For this review, take the finished solid that the model builds, in its own axes (mm). A direction names the side the tool comes from. Round coordinates to 2 decimals unless told otherwise and drop trailing zeros. Write each loop counter-clockwise with the first axis right and the second up, starting at its lowest first coordinate (ties: lowest second). Pieces come first, ordered by that corner, then holes. Notation, with made-up numbers: (68, 61.25) -> (91, 61.25) arc R12 ccw to (91, 68.25) -> close; hole circle Ø10 at (60, 75.25). An arc over 180 degrees is marked (long way). Answer as CSV lines item,"result". Start each with the question number.
Item 1: Take a section at C-C on y = 28. Give the boundary of the cut face in (x, z), then the cut area to 3 significant figures.
Item 2: Wall thickness on probe 1 along X at (y, z) = (23.5, -11.5); probe 2 along Y at (x, z) = (-25.5, 11.5); probe 3 along Z at (x, y) = (13, 22): over which ranges is each line inside the solid? List them lowest first. Write a range as from..to.
Item 3: Take a section at B-B on z = 19. Give the boundary of the cut face in (x, y), then the cut area to 3 significant figures.
Item 4: Take a section at A-A on z = -12.5. Give the boundary of the cut face in (x, y), then the cut area to 3 significant figures.
Item 5: Machinability: for faces 4 (the flat face through (-31, 2, -18.85)), 5 (the flat face through (-1, 5, -3)), 6 (the flat face through (18, 18, -16.85)), 7 (the flat face through (-1, 2, 21.15)), 8 (the cylindrical face through (-33.25, 2.54, 18.15)), which of the approach directions +Z, -Z, +X, -X, +Y, -Y give a long, thin tool a straight path to every point of the face, cutting with its end or side? Answer none if there is none.
Item 6: Take a section at D-D on x = -28. Give the boundary of the cut face in (y, z), then the cut area to 3 significant figures.
Item 7: For pin 1 Ø12 at (y, z) = (29, -4.5) entering from -X; pin 2 Ø13.5 at (y, z) = (20.5, -5) entering from +X; pin 3 Ø1.5 at (x, y) = (-7, 2.5) entering from +Z; pin 4 Ø6 at (y, z) = (20.5, -21) entering from +X, all flat-tipped, find the tip position at first contact; note any pin that passes through.
Item 8: Mouldability with a two-part tool opening along Z and no side actions: class faces 1 (the flat face through (31.289, 3, 1)), 2 (the flat face through (43.289, 2, 8)), 3 (the flat face through (-1, 20, 22.08)) as +Z half, -Z half, draft (parallel to the pull), parting line (faces both ways), or undercut.
```python
from build123d import *

# Parameters (mm, degrees)
EXTRUDE_1_DEPTH     = 5
SKETCH_4_W          = 1.8
SKETCH_4_H          = 37
EXTRUDE_2_DEPTH     = 27
SKETCH_5_W          = 40.5
SKETCH_5_H          = 37
EXTRUDE_3_DEPTH     = 3
CUT_EXTRUDE_4_DEPTH = 10
CUT_EXTRUDE_7_DEPTH = 10
CUT_EXTRUDE_8_DEPTH = 10
SKETCH_13_R         = 7.5
CUT_EXTRUDE_9_DEPTH = 10
SKETCH_14_W         = 40.5
SKETCH_14_H         = 30
EXTRUDE_4_DEPTH     = 2


with BuildPart() as part:
    # 草图1 → 凸台-拉伸1 (new body)
    with BuildSketch(Plane(origin=(0, 0, 0), x_dir=(1, 0, 0), z_dir=(0, 1, 0))):
        Polygon((13.545654436, 26.428234879), (-13.545654436, 26.428234879), (-19.229145808, 18.850246383), (-43.289259281, 18.850246383), (-43.289259281, -21.149753617), (43.289259281, -21.149753617), (43.289259281, 18.850246383), (19.229145808, 18.850246383), align=None)
    extrude(amount=EXTRUDE_1_DEPTH)

    # 草图4 → 凸台-拉伸2 (add)
    with BuildSketch(Plane(origin=(0, 5, 0), x_dir=(1, 0, 0), z_dir=(0, 1, 0))):
        with Locations((-20.389259281, -1.649753617)):
            Rectangle(SKETCH_4_W, SKETCH_4_H)
        with Locations((18.410740719, -1.649753617)):
            Rectangle(SKETCH_4_W, SKETCH_4_H)
    extrude(amount=EXTRUDE_2_DEPTH)

    # 草图5 → 凸台-拉伸3 (add)
    with BuildSketch(Plane(origin=(0, 32, 0), x_dir=(1, 0, 0), z_dir=(0, 1, 0))):
        with Locations((-0.939259281, -1.580342136)):
            Rectangle(SKETCH_5_W, SKETCH_5_H)
    extrude(amount=EXTRUDE_3_DEPTH)

    # 草图8 → 切除-拉伸4 (cut)
    with BuildSketch(Plane(origin=(0, 5, 0), x_dir=(1, 0, 0), z_dir=(0, 1, 0))):
        with BuildLine():
            Line((-31.289259281, 13.850246383), (-31.289259281, -16.149753617))
            ThreePointArc((-31.289259281, -16.149753617), (-33.289259281, -18.149753617), (-35.289259281, -16.149753617))
            Line((-35.289259281, -16.149753617), (-35.289259281, 13.850246383))
            ThreePointArc((-35.289259281, 13.850246383), (-33.289259281, 15.850246383), (-31.289259281, 13.850246383))
        make_face()
    extrude(amount=-CUT_EXTRUDE_4_DEPTH, mode=Mode.SUBTRACT)

    # 草图10 → 切除-拉伸7 (cut)
    with BuildSketch(Plane(origin=(0, 5, 0), x_dir=(1, 0, 0), z_dir=(0, 1, 0))):
        with BuildLine():
            Line((35.289259281, 13.850246383), (35.289259281, -16.149753617))
            ThreePointArc((35.289259281, -16.149753617), (33.289259281, -18.149753617), (31.289259281, -16.149753617))
            Line((31.289259281, -16.149753617), (31.289259281, 13.850246383))
            ThreePointArc((31.289259281, 13.850246383), (33.289259281, 15.850246383), (35.289259281, 13.850246383))
        make_face()
    extrude(amount=-CUT_EXTRUDE_7_DEPTH, mode=Mode.SUBTRACT)

    # 草图12 → 切除-拉伸8 (cut)
    with BuildSketch(Plane(origin=(0, 5, 0), x_dir=(1, 0, 0), z_dir=(0, 1, 0))):
        with BuildLine():
            Line((44.805959338, 6.484665103), (34.19935762, -4.121936615))
            ThreePointArc((34.19935762, -4.121936615), (32.785144058, -4.121936615), (32.785144058, -2.707723053))
            Line((32.785144058, -2.707723053), (43.391745776, 7.898878665))
            ThreePointArc((43.391745776, 7.898878665), (44.805959338, 7.898878665), (44.805959338, 6.484665103))
        make_face()
        with BuildLine():
            Line((-44.526375344, 6.888037873), (-33.523218079, -3.306594549))
            ThreePointArc((-33.523218079, -3.306594549), (-33.469316423, -4.719780528), (-34.882502402, -4.773682184))
            Line((-34.882502402, -4.773682184), (-45.885659667, 5.420950238))
            ThreePointArc((-45.885659667, 5.420950238), (-45.939561323, 6.834136217), (-44.526375344, 6.888037873))
        make_face()
    extrude(amount=-CUT_EXTRUDE_8_DEPTH, mode=Mode.SUBTRACT)

    # 草图13 → 切除-拉伸9 (cut)
    with BuildSketch(Plane(origin=(0, 35, 0), x_dir=(1, 0, 0), z_dir=(0, 1, 0))):
        with Locations((-0.989259281, -1.580342136)):
            Circle(SKETCH_13_R)
    extrude(amount=-CUT_EXTRUDE_9_DEPTH, mode=Mode.SUBTRACT)

    # 草图14 → 凸台-拉伸4 (add)
    with BuildSketch(Plane.XY.offset(20.080342136)):
        with Locations((-0.939259281, 20)):
            Rectangle(SKETCH_14_W, SKETCH_14_H)
    extrude(amount=EXTRUDE_4_DEPTH)


solid = part.part
```
Output values:
1,outline,"(-21.29, -16.85) -> (-19.49, -16.85) -> (-19.49, 20.08) -> (17.51, 20.08) -> (17.51, -16.85) -> (19.31, -16.85) -> (19.31, 22.08) -> (-21.19, 22.08) -> (-21.19, 20.15) -> (-21.29, 20.15) -> close"
1,area,"214 mm^2"
2,probe 1,"x = -21.29..-19.49, 17.51..19.31"
2,probe 2,"y = 0..5"
2,probe 3,"z = 20.08..22.08"
3,outline,"(-43.29, 0) -> (43.29, 0) -> (43.29, 5) -> (19.31, 5) -> (19.31, 35) -> (-21.19, 35) -> (-21.19, 32) -> (-21.29, 32) -> (-21.29, 5) -> (-43.29, 5) -> close; hole (-19.49, 5) -> (17.51, 5) -> (17.51, 32) -> (-19.49, 32) -> close"
3,area,"652 mm^2"
4,outline,"(-43.29, 0) -> (-35.29, 0) -> (-35.29, 5) -> (-43.29, 5) -> close; (-31.29, 0) -> (31.29, 0) -> (31.29, 5) -> (19.31, 5) -> (19.31, 35) -> (-21.19, 35) -> (-21.19, 32) -> (-21.29, 32) -> (-21.29, 5) -> (-31.29, 5) -> close; (35.29, 0) -> (43.29, 0) -> (43.29, 5) -> (35.29, 5) -> close; hole (-19.49, 5) -> (17.51, 5) -> (17.51, 32) -> (-19.49, 32) -> close"
4,area,"612 mm^2"
5,face 4,"-Z, -X, +Y, -Y"
5,face 5,"-Z"
5,face 6,"-Z, +X, -X"
5,face 7,"+Z, +X, -X, -Y"
5,face 8,"+Y, -Y"
6,outline,"(0, -18.85) -> (5, -18.85) -> (5, 21.15) -> (0, 21.15) -> close"
6,area,"200 mm^2"
7,pin 1,"stops at x = -21.29"
7,pin 2,"stops at x = 19.31"
7,pin 3,"stops at z = 21.15"
7,pin 4,"passes through"
8,face 1,"undercut"
8,face 2,"draft"
8,face 3,"+Z half"
